Work out the finished part from the listing and answer in its coordinate system (mm). A direction names the side the tool comes from. Round coordinates to 2 decimals unless told otherwise and drop trailing zeros. Order: outer loops, then holes, each group sorted by start corner. A loop starts at its lowest first (then second) coordinate and runs counter-clockwise, first axis right, second up. Notation, with made-up numbers: (25.5, -39.75) -> (66.5, -39.75) arc R20 ccw to (66.5, -11.75) -> close; hole circle Ø2 at (26.25, -6). An arc over 180 degrees is marked (long way). Use one line per item in the form item = value.
```python
from build123d import *

# Parameters (mm, degrees)
F1_DEPTH = 30
F2_R     = 7.3564369941
F3_DEPTH = 10.4896114323
F4_R     = 4.9643455943
F5_DEPTH = 137.8729965196
F7_DEPTH = 254
F8_DEPTH = 133.196592753


with BuildPart() as f1:
    # F0 (on Front) → F1 (new body)
    with BuildSketch(Plane.XZ):
        Polygon((1.0179836117, 36.3313048123), (-3.9518002313, 35.7824436691), (0, 0), (49.6978384293, 5.4886114323), (134.6978384293, 5.4886114323), (134.6978384293, 10.4886114323), (49.6978384293, 10.4886114323), (4.4242395946, 5.4886114323), align=None)
    extrude(amount=F1_DEPTH)

    # F2 (on face) → F3 (cut, through all)
    with BuildSketch(Plane.XY.offset(10.4886114323)):
        with Locations((90.8175626415, -15)):
            Circle(F2_R)
    extrude(amount=-F3_DEPTH, mode=Mode.SUBTRACT)

    # F4 (on face) → F5 (cut, through all)
    with BuildSketch(Plane(origin=(0, 0, 0), x_dir=(0, -1, 0), z_dir=(-0.9939567686, 0, -0.1097722286))):
        with Locations((15, 20.9979638457)):
            Circle(F4_R)
    extrude(amount=-F5_DEPTH, mode=Mode.SUBTRACT)

    # F6 (on face) → F7 (join, symmetric)
    with BuildSketch(Plane.XZ.offset(30)):
        Polygon((27.710283177, 39.2791927926), (1.0179836117, 36.3313048123), (4.4242395946, 5.4886114323), (31.1165391599, 8.4364994126), align=None)
        Polygon((8.8451622943, 11.0072564185), (6.5366285978, 31.9103821126), (23.2893604773, 33.7605478064), (25.5978941738, 12.8574221123), align=None, mode=Mode.SUBTRACT)
    extrude(amount=F7_DEPTH, both=True)

    # F8 (cut, through all): a face of the model
    f8_faces = [f1.faces().sort_by_distance(p)[0] for p in [
        (2.6647905545, -15, 21.4199294342),
    ]]
    extrude(f8_faces, amount=-F8_DEPTH, mode=Mode.SUBTRACT)


solid = f1.part
```
Item 1: The part is cut by section A-A, the plane y = 13.5. Give the vertices of the cut face in (x, z).
Findings:
outline = (1.02, 36.33) -> (4.42, 5.49) -> (31.12, 8.44) -> (27.71, 39.28) -> close; hole (6.54, 31.91) -> (8.85, 11.01) -> (25.6, 12.86) -> (23.29, 33.76) -> close
Item 2: For faces 1 (the flat face through (17.339, -33.556, 11.945)), 2 (the flat face through (40.537, -14.79, 9.477)), 3 (the flat face through (102, -15, 10.489)), 4 (the flat face through (82, -15, 5.489)), determine the directions among +Z, -Z, +X, -X, +Y, -Y from which every point of the face is accessible in a straight line to the end or side of a thin tool.
Findings:
face_1 = +Y, -Y
face_2 = +Z, +Y, -Y
face_3 = +Z, +X, +Y, -Y
face_4 = -Z, +X, +Y, -Y
Item 3: The part is cut by section B-B, the plane x = 125. Give the vertices of the cut face in (y, z), and give its area (3 significant figures).
Findings:
outline = (-30, 5.49) -> (0, 5.49) -> (0, 10.49) -> (-30, 10.49) -> close
area = 150 mm^2
Item 4: Consider line 1 along Z through (x, y) = (119, -19); line 2 along Z through (x, y) = (23, 179.5); line 3 along Z through (x, y) = (22, 79.5). Determine where each line is inside the solid, lowest interval first.
Findings:
line_1 = 5.49 to 10.49
line_2 = 7.54 to 12.57, 33.73 to 38.76
line_3 = 7.43 to 12.46, 33.62 to 38.65
Item 5: Determine the mould class of faces 5 (the flat face through (29.437, -33.556, 23.642)), 6 (the flat face through (7.707, -33.556, 21.312)), 7 (the flat face through (2.7, 110.4, 21.1)), 8 (the flat face through (55, -30, 10)) for opening direction Z: released by +Z, released by -Z, zero draft, split by the parting line, or undercut.
Findings:
face_5 = released by +Z
face_6 = undercut
face_7 = released by -Z
face_8 = zero draft
Item 6: Flat-ended cylindrical pins translate along their axes: P1, Ø6, axis at y = -153, z = 13.5, coming from the +X side; P2, Ø10, axis at x = 56, z = 18, coming from the +Y side; P3, Ø6, axis at y = 123.5, z = 4, coming from the -X side; P4, Ø5, axis at y = 9, z = 17.5, coming from the -X side. Find the tip coordinate at first contact, or state that the pin passes through.
Findings:
P1 = 30.89
P2 = through
P3 = 4.26
P4 = 2.82
